Can you work these out from the model? Positions are in its coordinate system, mm. A direction names the side the tool comes from. Give positions to 0.01 mm unless a question says otherwise; leave off trailing zeros. Loops run counter-clockwise (first coordinate to the right, second up) from the corner with the lowest first, then second, coordinate; pieces in that order, holes last. Notation, with made-up numbers: (61.5, 13) - (117.5, 13) arc R8 cw to (117.5, 23) - close; hole circle Ø4 at (-3, 76). An arc over 180 degrees is marked (long way). Answer as a JSON object with one key per item and string values. Group by question number.
Item 1: Suppose I cut it at B-B on z = -89. Write out the boundary of the cut face in (x, y).
Item 2: Thinking about a two-plate mould opening in Z: for faces 1 (the flat face through (-30, 26, -58)), 2 (the cylindrical face through (-45.297, 12.818, -6.014)), 3 (the cylindrical face through (-28.39, 164.48, -174.58)), 4 (the cylindrical face through (-39.872, 13.182, -15.386)), which applies, pulls with the +Z half, pulls with the -Z half, needs draft (parallel to the pull), parting line crosses it, or undercut?
Item 3: Suppose I cut it at A-A on x = -35.5. Write out the boundary of the cut face in (y, z), and give its area (3 significant figures).
Item 4: Will these pins go through, and if not, where does the flat tip stop? pin 1 (10 mm diameter, centred on x = -6, z = -25, fed in from -Y); pin 2 (8 mm diameter, centred on x = 15, y = 152, fed in from -Z); pin 3 (23 mm diameter, centred on x = 31, z = -89, fed in from +Y); pin 4 (3 mm diameter, centred on x = -15, y = 128.5, fed in from +Z).
Item 5: Please list where these lines run through material, in increasing order: L1, parallel to X at y = 7.25, z = -89; L2, parallel to Z at x = 34, y = 9.5; L3, parallel to Y at x = -42, z = -109.
Item 6: Which directions (+Z, -Z, +X, -X, +Y, -Y) give clear straight access to the entire face, cutting with the end or side of a thin tool? Please do faces 5 (the flat face through (10, 47, -88)), 6 (the cylindrical face through (0.8, 187.1, -201.9)), 7 (the flat face through (-10, 47, -88)).
Item 7: Suppose I cut it at D-D on y = 59.5. Write out the boundary of the cut face in (x, z).
Item 8: Suppose I cut it at C-C on y = 14. Write out the boundary of the cut face in (x, z), and give its area (3 significant figures).
from build123d import *

# Parameters (mm, degrees)
BOSS_EXTRUDE1_DEPTH = 51
CUT_EXTRUDE1_DEPTH  = 102
BOSS_EXTRUDE2_START = -26
SKETCH4_R           = 32
BOSS_EXTRUDE2_DEPTH = 60
SKETCH5_R           = 18.5
CUT_EXTRUDE2_DEPTH  = 316.950756304
BOSS_EXTRUDE3_DEPTH = 10
SKETCH7_R           = 10
CUT_EXTRUDE3_DEPTH  = 313.368418834
FILLET1_R           = 20


with BuildPart() as part:
    # Sketch2 → Boss-Extrude1 (new, symmetric)
    with BuildSketch(Plane(origin=(0, 0, 0), x_dir=(0, 0, -1), z_dir=(1, 0, 0))):
        Polygon((0, 0), (54.31624891, 0), (129, 0), (244.5, 200.051868274), (221.983339502, 213.051868274), (113.988893001, 26), (0, 26), align=None)
    extrude(amount=BOSS_EXTRUDE1_DEPTH, both=True)

    # Sketch3 → Cut-Extrude1 (cut)
    with BuildSketch(Plane(origin=(0, -42.858638544, -74.233339502), x_dir=(1, 0, 0), z_dir=(0, 0.49999999999999784, 0.86602540378444))):
        with BuildLine():
            Line((-51, 295.5), (-51, 244.5))
            ThreePointArc((-51, 244.5), (-36.062445841, 280.562445841), (0, 295.5))
            Line((0, 295.5), (-51, 295.5))
        make_face()
        with BuildLine():
            Line((51, 295.5), (0, 295.5))
            ThreePointArc((0, 295.5), (36.062445841, 280.562445841), (51, 244.5))
            Line((51, 244.5), (51, 295.5))
        make_face()
    extrude(amount=-CUT_EXTRUDE1_DEPTH, mode=Mode.SUBTRACT)

    # Sketch4 → Boss-Extrude2 (add)
    with BuildSketch(Plane(origin=(0, -42.858638544, -74.233339502), x_dir=(1, 0, 0), z_dir=(0, 0.49999999999999784, 0.86602540378444)).offset(BOSS_EXTRUDE2_START)):
        with Locations(Location((0, 244.5, 0), (0, 0, 270))):
            Circle(SKETCH4_R)
    extrude(amount=BOSS_EXTRUDE2_DEPTH)

    # Sketch5 → Cut-Extrude2 (cut, through all)
    with BuildSketch(Plane(origin=(0, -25.858638544, -44.788475772), x_dir=(1, 0, 0), z_dir=(0, 0.49999999999999784, 0.86602540378444))):
        with Locations(Location((0, 244.5, 0), (0, 0, 270))):
            Circle(SKETCH5_R)
    extrude(amount=-CUT_EXTRUDE2_DEPTH, mode=Mode.SUBTRACT)

    # Sketch6 → Boss-Extrude3 (add, symmetric)
    with BuildSketch(Plane(origin=(0, 0, 0), x_dir=(0, 0, -1), z_dir=(1, 0, 0))):
        Polygon((0, 26), (151.988893001, 91.817930688), (113.988893001, 26), align=None)
    extrude(amount=BOSS_EXTRUDE3_DEPTH, both=True)

    # Sketch7 → Cut-Extrude3 (cut, through all)
    with BuildSketch(Plane(origin=(0, 26, 0), x_dir=(1, 0, 0), z_dir=(0, 1, 0))):
        with Locations(Location((31, 20, 0), (0, 0, 270))):
            Circle(SKETCH7_R)
        with Locations(Location((-31, 20, 0), (0, 0, 270))):
            Circle(SKETCH7_R)
        with Locations(Location((-31, 89, 0), (0, 0, 270))):
            Circle(SKETCH7_R)
        with Locations(Location((31, 89, 0), (0, 0, 270))):
            Circle(SKETCH7_R)
    extrude(amount=-CUT_EXTRUDE3_DEPTH, mode=Mode.SUBTRACT)

    # Fillet1
    fillet1_edges = [part.edges().sort_by_distance(p)[0] for p in [
        (51, 13, 0),
        (-51, 13, 0),
    ]]
    fillet(fillet1_edges, radius=FILLET1_R)


solid = part.part
Worked out:
{
 "1": {"outline": "(-51, 0) - (-41, 0) - (-41, 26) - (-51, 26) - close; (-21, 0) - (21, 0) - (21, 26) - (10, 26) - (10, 64.54) - (-10, 64.54) - (-10, 26) - (-21, 26) - close; (41, 0) - (51, 0) - (51, 26) - (41, 26) - close"},
 "2": {"face 1": "needs draft", "face 2": "pulls with the +Z half", "face 3": "undercut", "face 4": "undercut"},
 "3": {"outline": "(0, -129) - (187.6, -237.31) - (200.6, -214.79) - (26, -113.99) - (26, -97.93) - (0, -97.93) - close; (0, -80.07) - (26, -80.07) - (26, -28.93) - (0, -28.93) - close; (0, -11.07) - (26, -11.07) - (26, -0.51) - (0, -0.51) - close", "area": "7,650 mm2"},
 "4": {"pin 1": "stops at y = 0", "pin 2": "stops at z = -217.98", "pin 3": "stops at y = 26", "pin 4": "stops at z = -172.3"},
 "5": {"L1": "x = -51 to -41, -21 to 21, 41 to 51", "L2": "z = -134.48 to -98.54, -79.46 to -29.54, -10.46 to -0.23", "L3": "y = 0 to 26"},
 "6": {"face 5": "+Z, +X, +Y", "face 6": "none", "face 7": "+Z, -X, +Y"},
 "7": {"outline": "(-51, -163.35) - (51, -163.35) - (51, -133.33) - (10, -133.33) - (10, -77.36) - (-10, -77.36) - (-10, -133.33) - (-51, -133.33) - close"},
 "8": {"outline": "(-51, -137.08) - (51, -137.08) - (51, -20) arc R20 ccw to (31, 0) - (-31, 0) arc R20 ccw to (-51, -20) - close; hole circle Ø20 at (-31, -89); hole circle Ø20 at (-31, -20); hole circle Ø20 at (31, -89); hole circle Ø20 at (31, -20)", "area": "12,600 mm2"}
}
